from build123d import *

# Parameters (mm, degrees)
SKETCH2_W           = 10
SKETCH2_H           = 2
SKETCH2_W_2         = 7
SKETCH2_H_2         = 34
BOSS_EXTRUDE1_DEPTH = 7
CUT_EXTRUDE1_REACH  = 91.384
SKETCH4_W           = 41.7
SKETCH4_H           = 4
SKETCH6_W           = 11.583545394
SKETCH6_H           = 3
SKETCH6_W_2         = 32.816454606
SKETCH6_W_3         = 7.183545394
SKETCH6_H_2         = 8.505079478
SKETCH6_R           = 1.9
SKETCH6_W_4         = 7.8
SKETCH6_H_3         = 9.292079478
BOSS_EXTRUDE2_DEPTH = 4
CHAMFER1_SIZE       = 5
CHAMFER2_SIZE       = 3
CHAMFER7_SIZE       = 2
SKETCH7_R           = 1.6
CUT_EXTRUDE2_DEPTH  = 3.5


with BuildPart() as part:
    # Sketch2 → Boss-Extrude1 (new body)
    with BuildSketch(Plane(origin=(0, -3.05, 0), x_dir=(1, 0, 0), z_dir=(0, 1, 0))):
        with Locations((74.3, -1)):
            Rectangle(SKETCH2_W, SKETCH2_H)
        Polygon((69.3, -2), (69.3, 0), (69.3, 4), (13.6, 4), (13.6, 0), (13.6, -2), (32.3, -2), (39.3, -2), align=None)
        with Locations((35.8, -19)):
            Rectangle(SKETCH2_W_2, SKETCH2_H_2)
        with Locations((8.6, -1)):
            Rectangle(SKETCH2_W, SKETCH2_H)
    extrude(amount=-BOSS_EXTRUDE1_DEPTH)

    # Cut-Extrude1: up to this face of the body (flat: up to its plane)
    cut_extrude1_end = Plane(part.part.faces().sort_by_distance((35.8, -6.55, 36))[0])
    # Sketch4 → Cut-Extrude1 (cut, up to the picked face)
    with BuildSketch(Plane(origin=(0, 0, -4), x_dir=(-1, 0, 0), z_dir=(0, 0, -1)), mode=Mode.PRIVATE) as cut_extrude1_sk1:
        with Locations((-41.45, -8.05)):
            Rectangle(SKETCH4_W, SKETCH4_H)
    cut_extrude1_tool1 = split(extrude(cut_extrude1_sk1.sketch, amount=-CUT_EXTRUDE1_REACH, mode=Mode.PRIVATE), bisect_by=cut_extrude1_end, keep=Keep.BOTH, mode=Mode.PRIVATE)
    add(cut_extrude1_tool1.solids().sort_by(Axis((41.45, -8.05, -4), (0, 0, 1)))[0], mode=Mode.SUBTRACT)

    # Sketch6 → Boss-Extrude2 (add)
    # profile 1 of 4: a face of its own
    with BuildSketch(Plane.XY.offset(36)):
        with Locations((26.508227303, -4.55)):
            Rectangle(SKETCH6_W, SKETCH6_H)
    # profile 2 of 4: a face of its own
    with BuildSketch(Plane.XY.offset(36)):
        with Locations((55.708227303, -4.55)):
            Rectangle(SKETCH6_W_2, SKETCH6_H)
    # profile 3 of 4: a face of its own
    with BuildSketch(Plane.XY.offset(36)):
        with Locations((75.708227303, -7.302539739)):
            Rectangle(SKETCH6_W_3, SKETCH6_H_2)
        with Locations((76.016454606, -7.655079478)):
            Circle(SKETCH6_R, mode=Mode.SUBTRACT)
    # profile 4 of 4: a face of its own
    with BuildSketch(Plane.XY.offset(36)):
        with Locations((16.816454606, -7.696039739)):
            Rectangle(SKETCH6_W_4, SKETCH6_H_3)
        with Locations((16.816454606, -8.442079478)):
            Circle(SKETCH6_R, mode=Mode.SUBTRACT)
    extrude(amount=-BOSS_EXTRUDE2_DEPTH)

    # Chamfer1
    chamfer1_edges = [part.edges().sort_by_distance(p)[0] for p in [
        (39.3, -4.55, 2),
        (32.3, -4.55, 2),
        (39.3, -4.55, 32),
        (32.3, -4.55, 32),
    ]]
    chamfer(chamfer1_edges, length=CHAMFER1_SIZE)

    # Chamfer2
    chamfer2_edges = [part.edges().sort_by_distance(p)[0] for p in [
        (72.116454606, -6.05, 34),
        (20.716454606, -6.05, 34),
    ]]
    chamfer(chamfer2_edges, length=CHAMFER2_SIZE)

    # Chamfer7
    chamfer7_edges = [part.edges().sort_by_distance(p)[0] for p in [
        (62.3, -6.05, -1),
        (20.6, -6.05, -1),
    ]]
    chamfer(chamfer7_edges, length=CHAMFER7_SIZE)
    chamfer7_2_edges = [part.edges().sort_by_distance(p)[0] for p in [
        (62.3, -10.05, -1),
        (20.6, -10.05, -1),
    ]]
    chamfer(chamfer7_2_edges, length=CHAMFER7_SIZE - 0.0001)  # a hair under: the kernel refuses the full size

    # Sketch7 → Cut-Extrude2 (cut)
    with BuildSketch(Plane(origin=(0, 0, 0), x_dir=(-1, 0, 0), z_dir=(0, 0, -1))):
        with Locations(Location((-74.3, -6.55, 0), (0, 0, 90))):
            Circle(SKETCH7_R)
        with Locations(Location((-8.6, -6.55, 0), (0, 0, 90))):
            Circle(SKETCH7_R)
    extrude(amount=-CUT_EXTRUDE2_DEPTH, mode=Mode.SUBTRACT)


solid = part.part
Part model, mm, in its own coordinate system. A direction names the side the tool comes from. Give positions to 0.01 mm unless a question says otherwise; leave off trailing zeros. Loops run counter-clockwise (first coordinate to the right, second up) from the corner with the lowest first, then second, coordinate; pieces in that order, holes last.
(1) Band-saw the part on C-C (x = 65). Write the cut outline in (y, z), and give its area (3 significant figures).
Return value:
outline: (-10.05, -4) - (-3.05, -4) - (-3.05, 2) - (-10.05, 2) - close; (-6.05, 32) - (-3.05, 32) - (-3.05, 36) - (-6.05, 36) - close
area: 54.0 mm2
(2) Band-saw the part on B-B (x = 75). Write the cut outline in (y, z).
Return value:
outline: (-11.56, 32) - (-9.26, 32) - (-9.26, 36) - (-11.56, 36) - close; (-10.05, 0) - (-7.99, 0) - (-7.99, 2) - (-10.05, 2) - close; (-6.05, 32) - (-3.05, 32) - (-3.05, 36) - (-6.05, 36) - close; (-5.11, 0) - (-3.05, 0) - (-3.05, 2) - (-5.11, 2) - close
(3) Pin check, flat tips, straight feed: pin 1 (2 mm diameter, centred on x = 10, y = -6.5, fed in from -Z); pin 2 (2.5 mm diameter, centred on y = -5, z = 20.5, fed in from +X); pin 3 (0.8 mm diameter, centred on y = -10, z = 35, fed in from -X). Stop position of each tip, or through.
Return value:
pin 1: stops at z = 0
pin 2: stops at x = 39.3
pin 3: stops at x = 12.92
(4) Pull direction X, two halves, no side cores. Call faces 4 (the flat face through (3.6, -7, 1)), 5 (the flat face through (21.59, -7.06, -1.04)), 6 (the flat face through (41.8, -4.5, 4.5)): pulls with the +X half, pulls with the -X half, needs draft (parallel to the pull), parting line crosses it, or undercut.
Return value:
face 4: pulls with the -X half
face 5: undercut
face 6: pulls with the +X half
(5) Band-saw the part on D-D (z = 21). Write the cut outline in (x, y), and give its area (3 significant figures).
Return value:
outline: (32.3, -6.05) - (39.3, -6.05) - (39.3, -3.05) - (32.3, -3.05) - close
area: 21.0 mm2
(6) Drill centre lines: line 1 along X through (y, z) = (-6.55, 1.25); line 2 along Z through (x, y) = (76, -6.25); line 3 along Z through (x, y) = (68, -8). Where is each one in solid material? Low to high.
Return value:
line 1: x = 3.6 to 7, 10.2 to 22.1, 60.8 to 72.7, 75.9 to 79.3
line 2: z = 0 to 2
line 3: z = -4 to 2
(7) Band-saw the part on A-A (x = 8.6). Write the cut outline in (y, z), and give its area (3 significant figures).
Return value:
outline: (-10.05, 0) - (-8.15, 0) - (-8.15, 2) - (-10.05, 2) - close; (-4.95, 0) - (-3.05, 0) - (-3.05, 2) - (-4.95, 2) - close
area: 7.60 mm2
(8) 3-axis set-ups, long thin cutter, end or side, ignore diameter. For faces 1 (the flat face through (41.8, -4.6, 29.5)), 2 (the flat face through (70.637, -7.571, 34.028)), 3 (the flat face through (22.195, -7.571, 34.028)): which of +Z, -Z, +X, -X, +Y, -Y reach the whole face in a straight line?
Return value:
face 1: +X, +Y, -Y
face 2: +Z, -Y
face 3: +Z, -Z, -Y
